Design review of the part built by this model. Coordinates are the model's own, in mm. Give positions to 0.01 mm unless a question says otherwise; leave off trailing zeros. Order: outer loops, then holes, each group sorted by start corner. A loop starts at its lowest first (then second) coordinate and runs counter-clockwise, first axis right, second up. Notation, with made-up numbers: M -32.5,53 L 20.5,53 A21 cw 20.5,66 Z; hole C 51.5,-8.5 d9. An arc over 180 degrees is marked long. Answer as a JSON object with one key per item and string values.
from build123d import *

# Parameters (mm, degrees)
F0_R     = 6.35
F1_DEPTH = 2.5
F2_R     = 3.2
F2_R_2   = 3.175
F3_DEPTH = 0.5


with BuildPart() as f1:
    # F0 (on Top) → F1 (new body)
    with BuildSketch(Plane.XY):
        Circle(F0_R)
    extrude(amount=F1_DEPTH)

    # F2 (on face) → F3 (cut)
    with BuildSketch(Plane.XY.offset(2.5)):
        Circle(F2_R)
        Circle(F2_R_2, mode=Mode.SUBTRACT)
    extrude(amount=-F3_DEPTH, mode=Mode.SUBTRACT)

    # F4 (on Front) → F5 (revolve)
    with BuildSketch(Plane.XZ):
        Polygon((0, 0), (-6.35, 0), (-4.5, -0.5), (0, -0.5), align=None)
    revolve(axis=Axis((0, 0, -0.25), (0, 0, -1)))


solid = f1.part
(1) Insertion check: pin 1 (1 mm diameter, centred on x = 5, y = 4, fed in from -Z). The pin has a flat end and moves straight along its axis. Give the tip position at first contact, or say it passes through.
Checked values:
{"pin 1": "stops at z = -0.12"}
(2) We need section A-A (y = 0). Write out the cut boundary in (x, z) (3 decimals).
Checked values:
{"outline": "M -6.35,0 L -4.5,-0.5 L 4.5,-0.5 L 6.35,0 L 6.35,2.5 L 3.2,2.5 L 3.2,2 L 3.175,2 L 3.175,2.5 L -3.175,2.5 L -3.175,2 L -3.2,2 L -3.2,2.5 L -6.35,2.5 Z"}
(3) We need section C-C (z = 1.55). Write out the cut boundary in (x, y).
Checked values:
{"outline": "C 0,0 d12.7"}
(4) To check wall thickness, follow L1, parallel to Z at x = 0.25, y = -5.5; L2, parallel to Z at x = -1.25, y = 5.25; L3, parallel to X at y = -1.75, z = 0.6. State the ranges of each line that lie inside material, in increasing order. Write a range as from..to.
Checked values:
{"L1": "z = -0.23..2.5", "L2": "z = -0.26..2.5", "L3": "x = -6.1..6.1"}
